```python
from build123d import *

# Parameters (mm, degrees)
BOSS_EXTRUDE1_DEPTH = 30
CUT_EXTRUDE1_DEPTH  = 90.32223687


with BuildPart() as part:
    # Sketch1 → Boss-Extrude1 (new body)
    with BuildSketch(Plane.XY):
        with BuildLine():
            Line((0, -9.14322974), (-74.492069921, -9.14322974))
            ThreePointArc((-74.492069921, -9.14322974), (-83.635299661, 0), (-74.492069921, 9.14322974))
            Line((-74.492069921, 9.14322974), (0, 9.14322974))
            ThreePointArc((0, 9.14322974), (9.14322974, 0), (0, -9.14322974))
        make_face()
    extrude(amount=BOSS_EXTRUDE1_DEPTH)

    # Sketch2 → Cut-Extrude1 (cut, through all)
    with BuildSketch(Plane.XY.offset(30)):
        Polygon((-3.5, 2.020725942), (-3.5, -2.020725942), (0, -4.041451884), (3.5, -2.020725942), (3.5, 2.020725942), (0, 4.041451884), align=None)
    extrude(amount=-CUT_EXTRUDE1_DEPTH, mode=Mode.SUBTRACT)


solid = part.part
```
Source: CAD feature listing. Evaluate the final solid. Frame: model axes, mm. A direction names the side the tool comes from. Round coordinates to 2 decimals unless told otherwise and drop trailing zeros. Loops run counter-clockwise (first coordinate to the right, second up) from the corner with the lowest first, then second, coordinate; pieces in that order, holes last. Notation, with made-up numbers: M 21,-39 L 80,-39 A3 cw 80,-35 Z; hole C 75.5,81.5 d5. An arc over 180 degrees is marked long. Put each result on its own line as item: value.
(1) Access query for faces 4 (the face through (-83.633, -0.201, 14.79)), 5 (the face through (1.726, -3.045, 15.21)). Directions: +Z, -Z, +X, -X, +Y, -Y. A direction counts if a zero-diameter tool reaches every point of the face in a straight line with its end or side. Return the directions, or none.
Solutions:
face 4: +Z, -Z, -X
face 5: +Z, -Z
(2) Ray query, line 1 (X direction, y = 0.25, z = 17.5); line 2 (X direction, y = 2.5, z = 9); line 3 (X direction, y = -7.25, z = 21.25). Return the intervals inside material, ascending. Write a range as [from, to].
Solutions:
line 1: [-83.63, -3.5], [3.5, 9.14]
line 2: [-83.29, -2.67], [2.67, 8.79]
line 3: [-80.06, 5.57]
(3) Pull-direction query (X, two-part tool) for faces 1 (the face through (9.14, 0.2, 14.79)), 2 (the face through (-1.726, 3.045, 15.21)), 3 (the face through (-37, -9.143, 15)); classes: released by +X, released by -X, zero draft, split by the parting line, or undercut.
Solutions:
face 1: released by +X
face 2: undercut
face 3: zero draft
(4) Section B-B, the plane z = 22.5. Return loops of the section in (x, y), and give its area (3 significant figures).
Solutions:
outline: M -74.49,-9.14 L 0,-9.14 A9.14 ccw 0,9.14 L -74.49,9.14 A9.14 ccw Z; hole M -3.5,-2.02 L 0,-4.04 L 3.5,-2.02 L 3.5,2.02 L 0,4.04 L -3.5,2.02 Z
area: 1,580 mm²
(5) Section A-A, the plane y = 0. Return loops of the section in (x, z).
Solutions:
outline: M -83.64,0 L -3.5,0 L -3.5,30 L -83.64,30 Z; M 3.5,0 L 9.14,0 L 9.14,30 L 3.5,30 Z
(6) First-contact query: pin 1 (1 mm diameter, centred on y = 3, z = 13.5, fed in from -X); pin 2 (4 mm diameter, centred on y = 5, z = 25, fed in from -X); pin 3 (6 mm diameter, centred on y = -4.5, z = 25, fed in from +X). Flat tips, straight axial feed; report the tip coordinate or a pass-through.
Solutions:
pin 1: x = -83.29
pin 2: x = -83.13
pin 3: x = 9.02
(7) Section C-C, the plane y = -7.5. Return loops of the section in (x, z), and give its area (3 significant figures).
Solutions:
outline: M -79.72,0 L 5.23,0 L 5.23,30 L -79.72,30 Z
area: 2,550 mm²
